The listing builds one solid part. Answer for the finished solid, in the listing's coordinates (mm). Round coordinates to 2 decimals unless told otherwise and drop trailing zeros. Loops run counter-clockwise (first coordinate to the right, second up) from the corner with the lowest first, then second, coordinate; pieces in that order, holes last. Notation, with made-up numbers: (29, 43.25) - (56, 43.25) arc R21 cw to (56, 78.25) - close; hole circle Ø5 at (69.25, 68). An arc over 180 degrees is marked (long way). Write item = value, one per line. Start each with the question number.
1) Given pin 1 Ø1.8 at (x, z) = (58.5, 1.5) entering from -Y; pin 2 Ø1.8 at (x, y) = (182.63, 27.22) entering from +Z; pin 3 Ø2 at (x, z) = (5.5, 2) entering from -Y; pin 4 Ø2 at (y, z) = (39.5, 0.5) entering from +X, each flat-ended and moving along its own axis, determine where each tip first touches the part or whether it passes through.
2) Section A-A, the plane z = 2.1 is taken. Determine the outline of the cut face in (x, y).
3) For a pull along Y with two mould halves and no side action, classify faces 1 (the cylindrical face through (198.34, 1.05, 1.73)), 2 (the flat face through (170.51, 42.17, 1.73)), 3 (the flat face through (157.365, 19.957, 1.726)), 4 (the flat face through (104, 59, 0)) as released by +Y, released by -Y, zero draft, split by the parting line, or undercut.
4) Straight lines are drawn through the part: line 1 along Y through (x, z) = (65, 2); line 2 along X through (y, z) = (89.5, 2.7); line 3 along X through (y, z) = (65, 2.65). For each, find the intervals that lie inside material, in ascending order.
5) Section B-B, the plane x = 114.5 is taken. Determine the outline of the cut face in (y, z), and give its area (3 significant figures).
6) Section C-C, the plane y = 20.5 is taken. Determine the outline of the cut face in (x, z), and give its area (3 significant figures).
from build123d import *

# Parameters (mm, degrees)
SKETCH3_R           = 3.5
SKETCH3_R_2         = 1.5
BOSS_EXTRUDE1_DEPTH = 3.5
FILLET1_R           = 10
FILLET2_R           = 3
SKETCH4_R           = 1
CUT_EXTRUDE1_DEPTH  = 10


with BuildPart() as part:
    # Sketch3 → Boss-Extrude1 (new body)
    with BuildSketch(Plane.XY):
        with BuildLine():
            Line((5.559439508, 52.5), (0, 47.32233047))
            Line((0, 47.32233047), (-17.67766953, 65))
            Line((-17.67766953, 65), (-5.17766953, 77.5))
            Line((-5.17766953, 77.5), (59.884076231, 77.5))
            Line((59.884076231, 77.5), (62, 89.5))
            ThreePointArc((62, 89.5), (65, 92.017298894), (68, 89.5))
            Line((68, 89.5), (70.115923769, 77.5))
            Line((70.115923769, 77.5), (135.17766953, 77.5))
            Line((135.17766953, 77.5), (203.838834765, 8.838834765))
            ThreePointArc((203.838834765, 8.838834765), (203.838834765, -8.838834765), (186.161165235, -8.838834765))
            Line((186.161165235, -8.838834765), (124.82233047, 52.5))
            Line((124.82233047, 52.5), (5.559439508, 52.5))
        make_face()
        with Locations((195, 0)):
            Circle(SKETCH3_R, mode=Mode.SUBTRACT)
        with Locations((0, 65)):
            Circle(SKETCH3_R_2, mode=Mode.SUBTRACT)
        with Locations((65, 65)):
            Circle(SKETCH3_R_2, mode=Mode.SUBTRACT)
        with Locations((65, 89.5)):
            Circle(SKETCH3_R_2, mode=Mode.SUBTRACT)
    extrude(amount=BOSS_EXTRUDE1_DEPTH)

    # Fillet1
    fillet1_edges = [part.edges().sort_by_distance(p)[0] for p in [
        (5.559439508, 52.5, 1.75),
        (-5.17766953, 77.5, 1.75),
        (135.17766953, 77.5, 1.75),
        (124.82233047, 52.5, 1.75),
    ]]
    fillet(fillet1_edges, radius=FILLET1_R)

    # Fillet2
    fillet2_edges = [part.edges().sort_by_distance(p)[0] for p in [
        (59.884076231, 77.5, 1.75),
        (70.115923769, 77.5, 1.75),
    ]]
    fillet(fillet2_edges, radius=FILLET2_R)

    # Sketch4 → Cut-Extrude1 (cut)
    with BuildSketch(Plane(origin=(0, 0, 0), x_dir=(-1, 0, 0), z_dir=(0, 0, -1))):
        with Locations((-167.776388924, 12.374368671)):
            Circle(SKETCH4_R)
        with Locations((-182.625631329, 27.223611076)):
            Circle(SKETCH4_R)
    extrude(amount=-CUT_EXTRUDE1_DEPTH, mode=Mode.SUBTRACT)


solid = part.part
Geometry check:
q1.pin_1 = 52.5
q1.pin_2 = through
q1.pin_3 = 51.16
q1.pin_4 = 174.18
q2.outline = (-17.68, 65) - (0, 47.32) - (2.68, 49.82) arc R10 cw to (9.49, 52.5) - (120.68, 52.5) arc R10 cw to (127.75, 49.57) - (186.16, -8.84) arc R12.5 ccw to (203.84, 8.84) - (138.11, 74.57) arc R10 ccw to (131.04, 77.5) - (72.63, 77.5) arc R3 cw to (69.68, 79.98) - (68, 89.5) arc R3.05 ccw to (62, 89.5) - (60.32, 79.98) arc R3 cw to (57.37, 77.5) - (-1.04, 77.5) arc R10 ccw to (-8.11, 74.57) - close; hole circle Ø3 at (0, 65); hole circle Ø3 at (65, 65); hole circle Ø3 at (65, 89.5); hole circle Ø2 at (167.78, 12.37); hole circle Ø2 at (182.63, 27.22); hole circle Ø7 at (195, 0)
q3.face_1 = undercut
q3.face_2 = released by +Y
q3.face_3 = released by -Y
q3.face_4 = zero draft
q4.line_1 = 52.5 to 63.5, 66.5 to 88, 91 to 92.02
q4.line_2 = 62 to 63.5, 66.5 to 68
q4.line_3 = -17.68 to -1.5, 1.5 to 63.5, 66.5 to 147.68
q5.outline = (52.5, 0) - (77.5, 0) - (77.5, 3.5) - (52.5, 3.5) - close
q5.area = 87.5 mm2
q6.outline = (156.82, 0) - (192.18, 0) - (192.18, 3.5) - (156.82, 3.5) - close
q6.area = 124 mm2
